The listing builds one solid part. Answer for the finished solid, in the listing's coordinates (mm). A direction names the side the tool comes from. Round coordinates to 2 decimals unless told otherwise and drop trailing zeros. Loops run counter-clockwise (first coordinate to the right, second up) from the corner with the lowest first, then second, coordinate; pieces in that order, holes last. Notation, with made-up numbers: (17, 6) -> (72, 6) arc R14 cw to (72, 11) -> close; hole circle Ø10 at (88.25, -17.75). An arc over 180 degrees is marked (long way). One line per question, with ' | ' between items.
from build123d import *

# Parameters (mm, degrees)
FILLET1_R          = 1
CHAMFER2_SIZE      = 0.5
CUT_EXTRUDE1_START = 4
CUT_EXTRUDE1_DEPTH = 128.428687888


# Read off the part's stored shape, not the designer's step: M10x1.0 Machine Threads Stud1
with BuildPart() as part:
    # Sketch1 → Revolve1 (revolve)
    with BuildSketch(Plane(origin=(0, 0, 0), x_dir=(1, 0, 0), z_dir=(0, 1, 0))):
        Polygon((0, 0), (0, -6), (46, -6), (46, -7.5), (106, -7.5), (106, -6), (131, -6), (131, 0), align=None)
    revolve(axis=Axis((0, 0, 0), (1, 0, 0)))

    # Fillet1
    fillet1_edges = [part.edges().sort_by_distance(p)[0] for p in [
        (106, 0, -6),
        (46, 0, -6),
    ]]
    fillet(fillet1_edges, radius=FILLET1_R)

    # M10x1.0 Machine Threads Stud1 outline → M10x1.0 Machine Threads Stud1 (revolve, cut)
    with BuildSketch(Plane.YX):
        with BuildLine():
            Line((6, 131), (4.4455, 131))
            Line((4.4455, 131), (5, 130.4455))
            Line((5, 130.4455), (5, 121))
            Line((5, 121), (4.580384758, 120.273205081))
            ThreePointArc((4.580384758, 120.273205081), (4.520444504, 120.128496508), (4.5, 119.973205081))
            Line((4.5, 119.973205081), (4.5, 119.373205081))
            ThreePointArc((4.5, 119.373205081), (4.675735931, 118.948941012), (5.1, 118.773205081))
            Line((5.1, 118.773205081), (6, 118.773205081))
            Line((6, 118.773205081), (6, 131))
        make_face()
    revolve(axis=Axis((0, 0, 0), (1, 0, 0)), mode=Mode.SUBTRACT)

    # Chamfer2
    chamfer2_edges = [part.edges().sort_by_distance(p)[0] for p in [
        (0, 0, -6),
    ]]
    chamfer(chamfer2_edges, length=CHAMFER2_SIZE)

    # Sketch3 → Cut-Extrude1 (cut, through all)
    with BuildSketch(Plane(origin=(0, 0, 0), x_dir=(1, 0, 0), z_dir=(0, 1, 0)).offset(CUT_EXTRUDE1_START)):
        with BuildLine():
            Line((-17, -2.5), (17, -2.5))
            ThreePointArc((17, -2.5), (19.5, 0), (17, 2.5))
            Line((17, 2.5), (-17, 2.5))
            Line((-17, 2.5), (-17, -2.5))
        make_face()
    extrude(amount=CUT_EXTRUDE1_DEPTH, mode=Mode.SUBTRACT)


solid = part.part
Q1. Given pin 1 Ø1.5 at (x, z) = (66, 6) entering from +Y; pin 2 Ø5 at (x, z) = (49.5, 3.5) entering from +Y; pin 3 Ø0.7 at (x, y) = (11.5, 5) entering from -Z, each flat-ended and moving along its own axis, determine where each tip first touches the part or whether it passes through.
Numbers:
pin 1: y = 5.36 | pin 2: y = 7.43 | pin 3: z = -3.79
Q2. A cutting plane is placed at D-D on x = 68. Give the vertices of the cut face in (y, z), plus the area to 3 significant figures.
Numbers:
outline: circle Ø15 at (0, 0) | area: 177 mm^2
Q3. For a pull along Z with two mould halves and no side action, classify faces 6 (the face through (76.42, -0.33, -7.493)), 7 (the face through (0, 0, 0)), 8 (the face through (10, 4, 0)) as pulls with the +Z half, pulls with the -Z half, needs draft (parallel to the pull), parting line crosses it, or undercut.
Numbers:
face 6: parting line crosses it | face 7: needs draft | face 8: undercut
Q4. Find the intervals of material crossed by line 1 (Z direction, x = 78, y = -4.5); line 2 (Z direction, x = 94, y = -5.5); line 3 (X direction, y = 4.75, z = 0), in increasing order. Write a range as from..to.
Numbers:
line 1: -6..6 | line 2: -5.1..5.1 | line 3: 19.5..118.89, 120.57..130.7
Q5. For faces 1 (the face through (19.5, 4.8, 0.1)), 2 (the face through (119.67, -0.59, 4.46)), 3 (the face through (131, 0, 0)), 4 (the face through (46, -2, -7)), 5 (the face through (112.969, -1.802, 5.723)), determine the directions among +Z, -Z, +X, -X, +Y, -Y from which every point of the face is accessible in a straight line to the end or side of a thin tool.
Numbers:
face 1: -X, +Y | face 2: none | face 3: +Z, -Z, +X, +Y, -Y | face 4: -X | face 5: +X
Q6. A cutting plane is placed at C-C on x = 22. Give the vertices of the cut face in (y, z), plus the area to 3 significant figures.
Numbers:
outline: circle Ø12 at (0, 0) | area: 113 mm^2
